The listing builds one solid part. Answer for the finished solid, in the listing's coordinates (mm). A direction names the side the tool comes from. Round coordinates to 2 decimals unless told otherwise and drop trailing zeros. Loops run counter-clockwise (first coordinate to the right, second up) from the corner with the lowest first, then second, coordinate; pieces in that order, holes last. Notation, with made-up numbers: M 50,-39 L 76,-39 A26 ccw 76,-7 Z; hole C 6,27.25 d2. An arc over 180 degrees is marked long. Answer as a JSON object with one key per item and string values.
```python
from build123d import *

# Parameters (mm, degrees)
ESTRUSIONE_ESTRUSIONE1_DEPTH = 1.5


with BuildPart() as part:
    # Schizzo1 → Estrusione-Estrusione1 (new body, symmetric)
    with BuildSketch(Plane(origin=(0, 0, 0), x_dir=(0, 0, -1), z_dir=(1, 0, 0))):
        Polygon((-46, -82.5), (-46, -43.5), (0, -43.5), (0, -40.5), (-46, -40.5), (-46, 40.5), (0, 40.5), (0, 43.5), (-46, 43.5), (-46, 82.5), (-27.6, 82.5), (-27.6, 85.5), (-9.2, 85.5), (-9.2, 82.5), (9.2, 82.5), (9.2, 85.5), (27.6, 85.5), (27.6, 82.5), (46, 82.5), (46, 1.5), (0, 1.5), (0, -1.5), (46, -1.5), (46, -82.5), (27.6, -82.5), (27.6, -85.5), (9.2, -85.5), (9.2, -82.5), (-9.2, -82.5), (-9.2, -85.5), (-27.6, -85.5), (-27.6, -82.5), align=None)
    extrude(amount=ESTRUSIONE_ESTRUSIONE1_DEPTH, both=True)


solid = part.part
```
Item 1: The part is cut by section C-C (z = 5). Give the vertices of the cut face in (x, y), then the cut area to 3 significant figures.
Values follow:
{"outline": "M -1.5,-82.5 L 1.5,-82.5 L 1.5,-43.5 L -1.5,-43.5 Z; M -1.5,-40.5 L 1.5,-40.5 L 1.5,40.5 L -1.5,40.5 Z; M -1.5,43.5 L 1.5,43.5 L 1.5,82.5 L -1.5,82.5 Z", "area": "477 mm^2"}
Item 2: The part is cut by section D-D (z = -17). Give the vertices of the cut face in (x, y).
Values follow:
{"outline": "M -1.5,-85.5 L 1.5,-85.5 L 1.5,-1.5 L -1.5,-1.5 Z; M -1.5,1.5 L 1.5,1.5 L 1.5,85.5 L -1.5,85.5 Z"}
Item 3: Determine the mould class of faces 4 (the face through (0, 84, -9.2)), 5 (the face through (0, -43.5, 23)), 6 (the face through (0, 84, 27.6)) for opening direction Z: released by +Z, released by -Z, zero draft, split by the parting line, or undercut.
Values follow:
{"face 4": "undercut", "face 5": "zero draft", "face 6": "released by +Z"}
Item 4: Flat-ended cylindrical pins translate along their axes: P1, Ø1.5, axis at x = 0, z = 34.5, coming from the -Y side; P2, Ø0.9, axis at x = 0.5, y = -42.5, coming from the +Z side; P3, Ø1.5, axis at x = 0, z = -3.5, coming from the +Y side. Find the tip coordinate at first contact, or state that the pin passes through.
Values follow:
{"P1": "y = -82.5", "P2": "z = 0", "P3": "y = 82.5"}
Item 5: The part is cut by section A-A (z = -34). Give the vertices of the cut face in (x, y), then the cut area to 3 significant figures.
Values follow:
{"outline": "M -1.5,-82.5 L 1.5,-82.5 L 1.5,-1.5 L -1.5,-1.5 Z; M -1.5,1.5 L 1.5,1.5 L 1.5,82.5 L -1.5,82.5 Z", "area": "486 mm^2"}
Item 6: Straight lines are drawn through the part: line 1 (Y direction, x = 1.3, z = 24); line 2 (Y direction, x = 0.9, z = 28); line 3 (Y direction, x = -0.1, z = -7). For each, find the intervals that lie inside material, in ascending order.
Values follow:
{"line 1": "-85.5 to -43.5, -40.5 to 40.5, 43.5 to 85.5", "line 2": "-82.5 to -43.5, -40.5 to 40.5, 43.5 to 82.5", "line 3": "-82.5 to -1.5, 1.5 to 82.5"}
Item 7: Which of the six approach directions +Z, -Z, +X, -X, +Y, -Y give full straight-line access (tool end or side, diameter ignored) to faces 1 (the face through (0, 84, -27.6)), 2 (the face through (0, -42, 0)), 3 (the face through (0, 0, 0))?
Values follow:
{"face 1": "-Z, +X, -X, +Y", "face 2": "+Z, +X, -X", "face 3": "-Z, +X, -X"}
